```python
from build123d import *

# Parameters (mm, degrees)
BOSS_EXTRUDE1_DEPTH     = 1186
SKETCH3_R               = 12.5
CUT_EXTRUDE1_DEPTH      = 18
CUT_EXTRUDE1_DEPTH_BACK = 18


with BuildPart() as part:
    # Sketch1 → Boss-Extrude1 (new body)
    with BuildSketch(Plane(origin=(0, 0, 0), x_dir=(1, 0, 0), z_dir=(0, 1, 0))):
        Polygon((-25, 25), (-5.958548116, 25), (-10, 18), (10, 18), (5.958548116, 25), (25, 25), (25, 5.958548116), (18, 10), (18, -10), (25, -5.958548116), (25, -25), (5.958548116, -25), (10, -18), (-10, -18), (-5.958548116, -25), (-25, -25), (-25, -5.958548116), (-18, -10), (-18, 10), (-25, 5.958548116), align=None)
    extrude(amount=BOSS_EXTRUDE1_DEPTH)

    # Sketch3 → Cut-Extrude1 (cut, two sides)
    with BuildSketch(Plane(origin=(0, 0, 0), x_dir=(0, 0, -1), z_dir=(1, 0, 0))) as cut_extrude1_sk:
        with Locations((0, 1136)):
            Circle(SKETCH3_R)
        with Locations((0, 1061)):
            Circle(SKETCH3_R)
        with Locations((0, 986)):
            Circle(SKETCH3_R)
        with Locations((0, 911)):
            Circle(SKETCH3_R)
        with Locations((0, 836)):
            Circle(SKETCH3_R)
        with Locations((0, 761)):
            Circle(SKETCH3_R)
        with Locations((0, 686)):
            Circle(SKETCH3_R)
        with Locations((0, 611)):
            Circle(SKETCH3_R)
        with Locations((0, 536)):
            Circle(SKETCH3_R)
        with Locations((0, 461)):
            Circle(SKETCH3_R)
        with Locations((0, 386)):
            Circle(SKETCH3_R)
        with Locations((0, 311)):
            Circle(SKETCH3_R)
        with Locations((0, 236)):
            Circle(SKETCH3_R)
        with Locations((0, 161)):
            Circle(SKETCH3_R)
        with Locations((0, 86)):
            Circle(SKETCH3_R)
        with Locations((0, 11)):
            Circle(SKETCH3_R)
        with Locations((0, -64)):
            Circle(SKETCH3_R)
        with Locations((0, -139)):
            Circle(SKETCH3_R)
        with Locations((0, -214)):
            Circle(SKETCH3_R)
        with Locations((0, -289)):
            Circle(SKETCH3_R)
        with Locations((0, -364)):
            Circle(SKETCH3_R)
        with Locations((0, -439)):
            Circle(SKETCH3_R)
        with Locations((0, -514)):
            Circle(SKETCH3_R)
    extrude(amount=CUT_EXTRUDE1_DEPTH, mode=Mode.SUBTRACT)
    extrude(cut_extrude1_sk.sketch, amount=-CUT_EXTRUDE1_DEPTH_BACK, mode=Mode.SUBTRACT)


solid = part.part
```
The listing builds one solid part. Answer for the finished solid, in the listing's coordinates (mm). A direction names the side the tool comes from. Give positions to 0.01 mm unless a question says otherwise; leave off trailing zeros. Write each loop counter-clockwise with the first axis right and the second up, starting at its lowest first coordinate (ties: lowest second). Pieces come first, ordered by that corner, then holes. Notation, with made-up numbers: M 76.5,13 L 128.5,13 A16 cw 128.5,23 Z; hole C 46,68 d2. An arc over 180 degrees is marked long. Write each question's results on one line, items separated by ' | '.
Q1. Consider L1, parallel to Z at x = -4.5, y = 150; L2, parallel to Z at x = 6.5, y = 338; L3, parallel to Z at x = 10.75, y = 161. Determine where each line is inside the solid, lowest interval first. Write a range as from..to.
Output values:
L1: -18..-5.94, 5.94..18 | L2: -25..-24.06, -18..18, 24.06..25 | L3: -25..-12.5, 12.5..25
Q2. Section A-A, the plane y = 124 is taken. Write down the section's boundary in (x, z).
Output values:
outline: M -25,-25 L -5.96,-25 L -10,-18 L 10,-18 L 5.96,-25 L 25,-25 L 25,-5.96 L 18,-10 L 18,10 L 25,5.96 L 25,25 L 5.96,25 L 10,18 L -10,18 L -5.96,25 L -25,25 L -25,5.96 L -18,10 L -18,-10 L -25,-5.96 Z
Q3. A flat-ended cylindrical pin translates along its axis: P1, Ø6, axis at x = 1.5, y = 829.5, coming from the +Z side. Find the tip coordinate at first contact, or state that the pin passes through.
Output values:
P1: z = 18
Q4. A tool of negligible diameter and unlimited length cuts with its end or side. For faces 1 (the flat face through (0, 1186, 0)), 2 (the cylindrical face through (0.25, 23.49, -0.46)), from which of +Z, -Z, +X, -X, +Y, -Y can it reach the whole face along a straight path? Write none if from no direction.
Output values:
face 1: +Z, -Z, +X, -X, +Y | face 2: none
Q5. For a pull along Z with two mould halves and no side action, classify faces 3 (the flat face through (0, 0, 15)), 4 (the flat face through (18, 723, 0)) as released by +Z, released by -Z, zero draft, split by the parting line, or undercut.
Output values:
face 3: zero draft | face 4: undercut
